For this review, take the finished solid that the model builds, in its own axes (mm). A direction names the side the tool comes from. Coordinates: 2 decimals unless noted, no trailing zeros. Loops run counter-clockwise (first coordinate to the right, second up) from the corner with the lowest first, then second, coordinate; pieces in that order, holes last. Notation, with made-up numbers: M -14.75,9.25 L 1.25,9.25 A6 cw 1.25,14.25 Z; hole C -33.75,86 d5. An arc over 180 degrees is marked long. Write each question's results on one line, items separated by ' | '. Start each with the question number.
```python
from build123d import *

# Parameters (mm, degrees)
CROQUIS2_W                         = 6
CROQUIS2_H                         = 12
BRIDA_BASE1_DEPTH                  = 1
BRIDA_DE_ARISTA1_STRIP_W           = 5.4732
BRIDA_DE_ARISTA1_STRIP_H           = 1
BRIDA_DE_ARISTA1_STRIP_CUT_DEPTH   = 12
BRIDA_DE_ARISTA1_STRIP_2_W         = 5.4732
BRIDA_DE_ARISTA1_STRIP_2_H         = 1
BRIDA_DE_ARISTA1_STRIP_CUT_2_DEPTH = 12
BRIDA_DE_ARISTA1_DEPTH             = 12
BRIDA_DE_ARISTA1_BEND_DEPTH        = 12
CROQUIS13_W                        = 2
CROQUIS13_H                        = 7
CORTAR_EXTRUIR1_DEPTH              = 10
CORTAR_EXTRUIR2_REACH              = 16.697
CROQUIS14_R                        = 1


# Sheet-metal steps are written as plain solids
with BuildPart() as part:
    # Croquis2 → Brida base1 (new body)
    with BuildSketch(Plane.XY):
        with Locations((3, 6)):
            Rectangle(CROQUIS2_W, CROQUIS2_H)
    extrude(amount=-BRIDA_BASE1_DEPTH)

    # Brida de arista1 strip (across the edge) → Brida de arista1 strip cut (cut)
    with BuildSketch(Plane(origin=(6, 12, -1), x_dir=(-1, 0, 0), z_dir=(0, -1, 0))):
        with Locations((-1, -0.5)):
            Rectangle(BRIDA_DE_ARISTA1_STRIP_W, BRIDA_DE_ARISTA1_STRIP_H)
    extrude(amount=BRIDA_DE_ARISTA1_STRIP_CUT_DEPTH, mode=Mode.SUBTRACT)

    # Brida de arista1 strip 2 (across the edge) → Brida de arista1 strip cut 2 (cut)
    with BuildSketch(Plane(origin=(0, 0, -1), x_dir=(1, 0, 0), z_dir=(0, 1, 0))):
        with Locations((-1, -0.5)):
            Rectangle(BRIDA_DE_ARISTA1_STRIP_2_W, BRIDA_DE_ARISTA1_STRIP_2_H)
    extrude(amount=BRIDA_DE_ARISTA1_STRIP_CUT_2_DEPTH, mode=Mode.SUBTRACT)

    # Brida de arista1 section (across the edge) → Brida de arista1 (add)
    with BuildSketch(Plane(origin=(6, 12, -1), x_dir=(-1, 0, 0), z_dir=(0, -1, 0))):
        with BuildLine():
            Line((0, 0.7366), (0, 5))
            Line((0, 5), (1, 5))
            Line((1, 5), (1, 0.7366))
            ThreePointArc((1, 0.7366), (1.215745145, 0.215745145), (1.7366, 0))
            Line((1.7366, 0), (1.7366, -1))
            ThreePointArc((1.7366, -1), (0.508638364, -0.491361636), (0, 0.7366))
        make_face()
    extrude(amount=BRIDA_DE_ARISTA1_DEPTH)

    # Brida de arista1 section 2 (across the edge) → Brida de arista1 bend (add)
    with BuildSketch(Plane(origin=(0, 0, -1), x_dir=(1, 0, 0), z_dir=(0, 1, 0))):
        with BuildLine():
            Line((0, 0.7366), (0, 5))
            Line((0, 5), (1, 5))
            Line((1, 5), (1, 0.7366))
            ThreePointArc((1, 0.7366), (1.215745145, 0.215745145), (1.7366, 0))
            Line((1.7366, 0), (1.7366, -1))
            ThreePointArc((1.7366, -1), (0.508638364, -0.491361636), (0, 0.7366))
        make_face()
    extrude(amount=BRIDA_DE_ARISTA1_BEND_DEPTH)

    # Croquis13 → Cortar-Extruir1 (cut)
    with BuildSketch(Plane(origin=(6, 0, 0), x_dir=(0, 0, -1), z_dir=(1, 0, 0))):
        with Locations((1, 8.5)):
            Rectangle(CROQUIS13_W, CROQUIS13_H)
    extrude(amount=-CORTAR_EXTRUIR1_DEPTH, mode=Mode.SUBTRACT)

    # Cortar-Extruir2: up to this face of the body (flat: up to its plane)
    cortar_extruir2_end = Plane(part.part.faces().sort_by_distance((0, 5.906533244, -3.943073405))[0])
    # Croquis14 → Cortar-Extruir2 (cut, up to the picked face)
    with BuildSketch(Plane(origin=(6, 0, 0), x_dir=(0, 0, -1), z_dir=(1, 0, 0)), mode=Mode.PRIVATE) as cortar_extruir2_sk1:
        with Locations((4, 10.3)):
            Circle(CROQUIS14_R)
    cortar_extruir2_tool1 = split(extrude(cortar_extruir2_sk1.sketch, amount=-CORTAR_EXTRUIR2_REACH, mode=Mode.PRIVATE), bisect_by=cortar_extruir2_end, keep=Keep.BOTH, mode=Mode.PRIVATE)
    add(cortar_extruir2_tool1.solids().sort_by(Axis((6, 10.3, -4), (-1, 0, 0)))[0], mode=Mode.SUBTRACT)


solid = part.part
```
Q1. Take a section at C-C, the plane z = -2.4. Give the boundary of the cut face in (x, y).
Q2. Take a section at A-A, the plane z = -4. Give the boundary of the cut face in (x, y), then the cut area to 3 significant figures.
Q3. Take a section at B-B, the plane y = 10.3. Give the boundary of the cut face in (x, z), then the cut area to 3 significant figures.
Q4. Insertion check: P1, Ø2, axis at y = 4.5, z = -3.5, coming from the -X side; P2, Ø1, axis at x = 2, z = -1, coming from the +Y side; P3, Ø1.1, axis at x = 0.5, y = 8, coming from the +Z side. Each pin has a flat end and moves straight along its axis. Give the tip position at first contact, or say it passes through.
Q5. The part is to be moulded in two halves that separate along Z. For faces 1 (the face through (5.5, 9.7, -3.2)), 2 (the face through (3, 3, 0)), 3 (the face through (3, 3, -1)), say which applies: pulls with the +Z half, pulls with the -Z half, needs draft (parallel to the pull), parting line crosses it, or undercut.
Q6. For faces 4 (the face through (0.5, 8.5, -2)), 5 (the face through (5, 6, -4)), 6 (the face through (5.5, 6.1, -6)), list the 3-axis set-ups (+Z, -Z, +X, -X, +Y, -Y) from which the entire face can be reached by the end or side of a thin tool; tool diameter is ignored.
Q7. Take a section at D-D, the plane y = 8.5. Give the boundary of the cut face in (x, z).
Q8. To check wall thickness, follow line 1 along X through (y, z) = (5, -3.65); line 2 along Y through (x, z) = (5.5, -4); line 3 along Y through (x, z) = (3.05, -0.25). State the ranges of each line that lie inside material, in increasing order.
Results:
1) outline: M 0,0 L 1,0 L 1,12 L 0,12 Z; M 5,0 L 6,0 L 6,12 L 5,12 Z
2) outline: M 0,0 L 1,0 L 1,9.3 L 0,9.3 Z; M 0,11.3 L 1,11.3 L 1,12 L 0,12 Z; M 5,0 L 6,0 L 6,9.3 L 5,9.3 Z; M 5,11.3 L 6,11.3 L 6,12 L 5,12 Z | area: 20.0 mm^2
3) outline: M 0,-6 L 1,-6 L 1,-5 L 0,-5 Z; M 0,-3 L 1,-3 L 1,-2 L 0,-2 Z; M 5,-6 L 6,-6 L 6,-5 L 5,-5 Z; M 5,-3 L 6,-3 L 6,-2 L 5,-2 Z | area: 4.00 mm^2
4) P1: x = 0 | P2: y = 5 | P3: z = -2
5) face 1: undercut | face 2: pulls with the +Z half | face 3: pulls with the -Z half
6) face 4: +Z, +X, -X, +Y | face 5: -Z, +Y, -Y | face 6: -Z, +X, -X, +Y, -Y
7) outline: M 0,-6 L 1,-6 L 1,-2 L 0,-2 Z; M 5,-6 L 6,-6 L 6,-2 L 5,-2 Z
8) line 1: 0 to 1, 5 to 6 | line 2: 0 to 9.3, 11.3 to 12 | line 3: 0 to 5
